```python
from build123d import *

# Parameters (mm, degrees)
BOSS_EXTRUDE1_DEPTH = 1.8
FILLET1_R           = 0.5
SKETCH2_R           = 1.75
BOSS_EXTRUDE3_DEPTH = 1.8
CUT_EXTRUDE2_DEPTH  = 1.8
FILLET2_R           = 0.5
FILLET3_R           = 3


with BuildPart() as part:
    # Sketch1 → Boss-Extrude1 (new body)
    with BuildSketch(Plane.XY):
        with BuildLine():
            Line((0, 4.5), (0, 6.5))
            Line((0, 6.5), (6, 6.5))
            Line((6, 6.5), (6, 10.5))
            Line((6, 10.5), (10, 14.5))
            Line((10, 14.5), (10, 83.5))
            Line((10, 83.5), (16.4, 83.5))
            ThreePointArc((16.4, 83.5), (17.2719581, 81.425344658), (17.601960582, 79.199226044))
            Line((17.601960582, 79.199226044), (18.25, 49.5))
            Line((18.25, 49.5), (12, 49.5))
            Line((12, 49.5), (12, 37))
            add(Edge.make_bspline(
                [(12, 37), (12, 35.742192932), (12.5, 34.153450807), (12.5, 32.15)],
                knots=[0, 0, 0, 0, 1, 1, 1, 1], degree=3))
            Line((12.5, 32.15), (12.5, 2.89))
            ThreePointArc((12.5, 2.89), (11.653538598, 0.846461402), (9.61, 0))
            ThreePointArc((9.61, 0), (4.304293167, 1.180712741), (0, 4.5))
        make_face()
    extrude(amount=BOSS_EXTRUDE1_DEPTH)

    # Fillet1
    fillet1_edges = [part.edges().sort_by_distance(p)[0] for p in [
        (0, 4.5, 0.9),
        (0, 6.5, 0.9),
        (6, 6.5, 0.9),
        (6, 10.5, 0.9),
        (10, 14.5, 0.9),
        (10, 83.5, 0.9),
        (18.25, 49.5, 0.9),
        (12, 49.5, 0.9),
    ]]
    fillet(fillet1_edges, radius=FILLET1_R)

    # Sketch2 → Boss-Extrude3 (add)
    with BuildSketch(Plane.XY):
        with BuildLine():
            Line((7, -2.499596966), (7, 0.500403034))
            Line((7, 0.500403034), (11, 0.500403034))
            Line((11, 0.500403034), (11.824045318, -1.578286292))
            ThreePointArc((11.824045318, -1.578286292), (9.968981185, -4.955214332), (7, -2.499596966))
        make_face()
        with Locations((9.5, -2.499596966)):
            Circle(SKETCH2_R, mode=Mode.SUBTRACT)
    extrude(amount=BOSS_EXTRUDE3_DEPTH)

    # Sketch5 → Cut-Extrude2 (cut)
    with BuildSketch(Plane.XY):
        Polygon((10, 29.542425494), (10, 3.09), (19.868157727, 3.09), (19.868157727, -10.013619472), (-11.195906999, -10.013619472), (-11.195906999, 29.542425494), align=None)
    extrude(amount=CUT_EXTRUDE2_DEPTH, mode=Mode.SUBTRACT)

    # Fillet2
    fillet2_edges = [part.edges().sort_by_distance(p)[0] for p in [
        (10, 3.09, 0.9),
        (12.5, 3.09, 0.9),
    ]]
    fillet(fillet2_edges, radius=FILLET2_R)

    # Fillet3
    fillet3_edges = [part.edges().sort_by_distance(p)[0] for p in [
        (16.4, 83.5, 0.9),
    ]]
    fillet(fillet3_edges, radius=FILLET3_R)


solid = part.part
```
Can you work these out from the model? Positions are in its coordinate system, mm. A direction names the side the tool comes from. Round coordinates to 2 decimals unless told otherwise and drop trailing zeros. Loops run counter-clockwise (first coordinate to the right, second up) from the corner with the lowest first, then second, coordinate; pieces in that order, holes last. Notation, with made-up numbers: (-3.75, -39) -> (37.25, -39) arc R32 ccw to (37.25, -1) -> close; hole circle Ø3 at (6.25, 17). An arc over 180 degrees is marked (long way). Answer in a Markdown table with one row per item.
Item 1: If I drill on probe 1 along Y at (x, z) = (12.75, 0.4); probe 2 along X at (y, z) = (48.5, 0.2); probe 3 along X at (y, z) = (12.5, 0.15), over which ranges is the centre line in solid material (lowest first)?
Answer block:
| item | result |
|---|---|
| probe 1 | 49.5 to 83.5 |
| probe 2 | 10 to 12 |
| probe 3 | 10 to 12.5 |
Item 2: On a 3-axis mill with a long thin cutter (end or side, diameter ignored), from which of +Z, -Z, +X, -X, +Y, -Y can I reach the whole of each face in a straight line? I mean faces 1 (the flat face through (12, 83.5, 1)), 2 (the flat face through (12.5, 18, 1)). Say none if no direction works.
Answer block:
| item | result |
|---|---|
| face 1 | +Z, -Z, +X, -X, +Y |
| face 2 | +Z, -Z, +X, -Y |
Item 3: Will these pins go through, and if not, where does the flat tip stop? P1, Ø0.9, axis at y = 44.5, z = 1, coming from the +X side; P2, Ø0.9, axis at y = 11.5, z = 0.5, coming from the +X side; P3, Ø4, axis at x = 15.5, y = 24, coming from the +Z side; P4, Ø1, axis at x = 17.5, z = 1, coming from the -Y side.
Answer block:
| item | result |
|---|---|
| P1 | x = 12 |
| P2 | x = 12.5 |
| P3 | through |
| P4 | y = 49.5 |
Item 4: We'd pull the mould along Y, two halves only. Please class faces 3 (the flat face through (10, 43, 1)), 4 (the cylindrical face through (17.518, 80.246, 0.887)), 5 (the flat face through (12, 43, 1)): released by +Y, released by -Y, zero draft, split by the parting line, or undercut.
Answer block:
| item | result |
|---|---|
| face 3 | zero draft |
| face 4 | released by +Y |
| face 5 | undercut |
Item 5: Suppose I cut it at A-A, the plane y = 9.5. List the corners of the cut face in (x, z) for me.
Answer block:
| item | result |
|---|---|
| outline | (10, 0) -> (12.5, 0) -> (12.5, 1.8) -> (10, 1.8) -> close |
Item 6: Suppose I cut it at B-B, the plane x = 15.75. List the corners of the cut face in (y, z) for me.
Answer block:
| item | result |
|---|---|
| outline | (49.5, 0) -> (83.19, 0) -> (83.19, 1.8) -> (49.5, 1.8) -> close |
